```python
from build123d import *

# Parameters (mm, degrees)
SKETCH1_R           = 13.668
SKETCH1_R_2         = 10.668
BOSS_EXTRUDE1_DEPTH = 20
SKETCH2_R           = 20
BOSS_EXTRUDE2_DEPTH = 4
SKETCH3_R           = 2
M4_DRILL_DEPTH      = 4


with BuildPart() as part:
    # Sketch1 → Boss-Extrude1 (new body)
    with BuildSketch(Plane.XY):
        Circle(SKETCH1_R)
        Circle(SKETCH1_R_2, mode=Mode.SUBTRACT)
    extrude(amount=BOSS_EXTRUDE1_DEPTH)

    # Sketch2 → Boss-Extrude2 (add)
    with BuildSketch(Plane(origin=(0, 0, 0), x_dir=(-1, 0, 0), z_dir=(0, 0, -1))):
        Circle(SKETCH2_R)
    extrude(amount=BOSS_EXTRUDE2_DEPTH)

    # Sketch3 → M4_DRILL (cut)
    with BuildSketch(Plane.XY):
        with Locations((0, 16.5)):
            Circle(SKETCH3_R)
        with Locations((16.5, 0)):
            Circle(SKETCH3_R)
        with Locations((0, -16.5)):
            Circle(SKETCH3_R)
        with Locations((-16.5, 0)):
            Circle(SKETCH3_R)
    extrude(amount=-M4_DRILL_DEPTH, mode=Mode.SUBTRACT)


solid = part.part
```
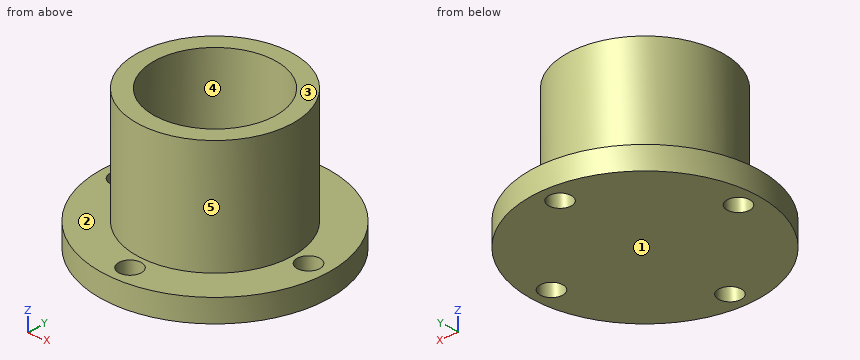
Work out the finished part from the listing and answer in its coordinate system (mm). Face numbers are marked on the shaded views. A direction names the side the tool comes from. Give positions to 0.01 mm unless a question says otherwise; leave off trailing zeros. Loops run counter-clockwise (first coordinate to the right, second up) from the corner with the lowest first, then second, coordinate; pieces in that order, holes last. Notation, with made-up numbers: M 81,1 L 99,1 A25 ccw 99,30 Z; hole C -6,68.25 d5. An arc over 180 degrees is marked long. One line per item, written item: value. Start each with the question number.
1. Find section A-A (y = 0). Give the vertices of the cut face in (x, z).
2. Which of the six approach directions +Z, -Z, +X, -X, +Y, -Y give full straight-line access (tool end or side, diameter ignored) to the marked faces 1 and 2?
3. Each of these flat-tipped pins is pushed along its axis until it touches: P1, Ø2, axis at y = -12.5, z = 15.5, coming from the +X side; P2, Ø1, axis at x = -7.5, z = 12, coming from the +Y side; P3, Ø8, axis at x = -15.5, z = 6.5, coming from the -Y side. Where does it stop, or does it pass through?
4. Determine the mould class of the marked faces 3, 4 and 5 for opening direction X: released by +X, released by -X, zero draft, split by the parting line, or undercut.
5. Find section C-C (x = 4). Give the vertices of the cut face in (y, z).
6. Find section B-B (x = -16.5). Give the vertices of the cut face in (y, z), and give its area (3 significant figures).
7. Find the intervals of material crossed by probe 1 along Y at (x, z) = (0, -1.3); probe 2 along Y at (x, z) = (0, 6.25); probe 3 along X at (y, z) = (6, 15.5), in increasing order.
Reported:
1. outline: M -20,-4 L -18.5,-4 L -18.5,0 L -20,0 Z; M -14.5,-4 L 14.5,-4 L 14.5,0 L 13.67,0 L 13.67,20 L 10.67,20 L 10.67,0 L -10.67,0 L -10.67,20 L -13.67,20 L -13.67,0 L -14.5,0 Z; M 18.5,-4 L 20,-4 L 20,0 L 18.5,0 Z
2. face 1: -Z, +X, -X, +Y, -Y
2. face 2: +Z
3. P1: stops at x = 7.39
3. P2: stops at y = 11.74
3. P3: stops at y = -7.39
4. face 3: zero draft
4. face 4: undercut
4. face 5: split by the parting line
5. outline: M -19.6,-4 L 19.6,-4 L 19.6,0 L 13.07,0 L 13.07,20 L 9.89,20 L 9.89,0 L -9.89,0 L -9.89,20 L -13.07,20 L -13.07,0 L -19.6,0 Z
6. outline: M -11.3,-4 L -2,-4 L -2,0 L -11.3,0 Z; M 2,-4 L 11.3,-4 L 11.3,0 L 2,0 Z
6. area: 74.4 mm²
7. probe 1: y = -20 to -18.5, -14.5 to 14.5, 18.5 to 20
7. probe 2: y = -13.67 to -10.67, 10.67 to 13.67
7. probe 3: x = -12.28 to -8.82, 8.82 to 12.28
